from build123d import *

# Parameters (mm, degrees)
F1_DEPTH = 6
F2_R     = 9
F3_R     = 4
F4_DEPTH = 25
F7_R     = 1.35
F8_DEPTH = 25


with BuildPart() as f1:
    # F0 (on Right) → F1 (new body)
    with BuildSketch(Plane.YZ):
        Polygon((-100, 0), (0, 0), (-49.4545935502, 18), (-100, 18), align=None)
    extrude(amount=F1_DEPTH)

    # F2
    f2_edges = [f1.edges().sort_by_distance(p)[0] for p in [
        (3, -100, 18),
    ]]
    fillet(f2_edges, radius=F2_R)

    # F3 (on face) → F4 (join)
    with BuildSketch(Plane.YZ.offset(6)):
        with Locations((-91, 9)):
            Circle(F3_R)
    extrude(amount=F4_DEPTH)


with BuildPart() as f5_1:
    # F5: instance of F1
    add(f1.part.mirror(Plane.YZ))

    # F7 (on face) → F8 (cut)
    with BuildSketch(Plane(origin=(0, 0, 0), x_dir=(1, 0, 0), z_dir=(0, 0.3420201433, 0.9396926208))):
        with Locations((-3, -45)):
            Circle(F7_R)
        with Locations((-3, -30)):
            Circle(F7_R)
    extrude(amount=-F8_DEPTH, mode=Mode.SUBTRACT)


solid = f5_1.part
The listing builds one solid part. Answer for the finished solid, in the listing's coordinates (mm). A direction names the side the tool comes from. Give positions to 0.01 mm unless a question says otherwise; leave off trailing zeros. Write each loop counter-clockwise with the first axis right and the second up, starting at its lowest first coordinate (ties: lowest second). Pieces come first, ordered by that corner, then holes.
1) Find the intervals of material crossed by L1, parallel to X at y = -96, z = 12.25; L2, parallel to Y at x = -29, z = 9.5; L3, parallel to Y at x = -25, z = 11.25, in increasing order.
2) For a pull along Z with two mould halves and no side action, classify faces 1 (the face through (-2.4, -46.3, 7.9)), 2 (the face through (-3.042, -97.294, 15.434)), 3 (the face through (-6, -62, 7)) as pulls with the +Z half, pulls with the -Z half, needs draft (parallel to the pull), parting line crosses it, or undercut.
3) Section C-C (y = -19) is taken. Write down the section's boundary in (x, z), and give its area (3 significant figures).
4) Section B-B (y = -63.5) is taken. Write down the section's boundary in (x, z), and give its area (3 significant figures).
5) Given P1, Ø4, axis at x = -19.5, z = 16, coming from the +Y side; P2, Ø4, axis at x = -25.5, z = 3.5, coming from the +Y side; P3, Ø2, axis at x = -8.5, z = 11, coming from the -Y side; P4, Ø1, axis at y = -68, z = 11.5, coming from the -X side, each flat-ended and moving along its own axis, determine where each tip first touches the part or whether it passes through.
6) Section A-A (x = -13.5) is taken. Write down the section's boundary in (y, z), and give its area (3 significant figures).
7) A tool of negligible diameter and unlimited length cuts with its end or side. For faces 4 (the face through (-2.958, -24.381, 8.874)), 5 (the face through (-18, -95, 9)), from which of +Z, -Z, +X, -X, +Y, -Y can it reach the whole face along a straight path? Write none if from no direction.
Response:
1. L1: x = -6 to 0
1. L2: y = -94.97 to -87.03
1. L3: y = -94.31 to -87.69
2. face 1: undercut
2. face 2: pulls with the +Z half
2. face 3: needs draft
3. outline: (-6, 0) - (0, 0) - (0, 6.92) - (-6, 6.92) - close
3. area: 41.5 mm2
4. outline: (-6, 0) - (0, 0) - (0, 18) - (-6, 18) - close
4. area: 108 mm2
5. P1: passes through
5. P2: stops at y = -89.06
5. P3: stops at y = -94.87
5. P4: stops at x = -6
6. outline: circle Ø8 at (-91, 9)
6. area: 50.3 mm2
7. face 4: +Z, +X, -X, +Y
7. face 5: -X
